Autodesk Inventor part; units mm, degrees
ref_plane "YZ Plane" through (0, 0, 0) normal (1, 0, 0) x (0, 1, 0)
ref_plane "XZ Plane" through (0, 0, 0) normal (0, 1, 0) x (-1, 0, 0)
ref_plane "XY Plane" through (0, 0, 0) normal (0, 0, 1) x (1, 0, 0)
sketch "Sketch1" plane through (0, 0, 0) normal (1, 0, 0) x (0, 1, 0)
  line L0 (0, 0) -> (50.8, 0)
  line L1 (50.8, 0) -> (50.8, -25.4)
  line L2 (50.8, -25.4) -> (0, -25.4)
  line L3 (0, -25.4) -> (0, 0)
  line L4 (47.625, -22.225) -> (47.625, -3.175)
  line L5 (47.625, -3.175) -> (3.175, -3.175)
  line L6 (3.175, -3.175) -> (3.175, -22.225)
  line L7 (3.175, -22.225) -> (47.625, -22.225)
  dimension "d0" = 50.8
  dimension "d1" = 25.4
  dimension "d2" = 3.175
extrude "Extrusion1" add sketch "Sketch1" along normal blind 177.8
sketch "Sketch2" plane through (0, 0, 0) normal (0, 0, 1) x (1, 0, 0)
  line L0 (0, 0) -> (0, 50.8)
  circle A0 centre (81.28, 25.4) radius 14.2875
  line L1 (151.13, 25.4) -> (175.8823, 25.4) construction
  line L2 (81.28, 25.4) -> (106.68, 25.4) construction
  circle A1 centre (99.2405, 43.3605) radius 2.0193
  circle A2 centre (63.3195, 7.4395) radius 2.0193
  circle A3 centre (63.3195, 7.4395) radius 2.0193
  circle A4 centre (99.2405, 43.3605) radius 2.0193
  dimension "d5" = 81.28
  dimension "d6" = 28.575
  dimension "d19" = 4.0386
  dimension "d20" = 4.0386
extrude "Extrusion2" cut sketch "Sketch2" against normal blind 25.4 contours A0
sketch "Sketch3" plane through (177.8, 0, 0) normal (1, 0, 0) x (0, 0, -1)
  line L0 (0, 50.8) -> (0, 0)
  line L1 (25.4, 0) -> (25.4, 50.8)
  line L2 (0, 0) -> (25.4, 0)
  line L3 (25.4, 0) -> (25.4, 50.8)
  line L4 (25.4, 50.8) -> (0, 50.8)
  line L5 (0, 50.8) -> (0, 0)
  line L6 (3.175, 3.175) -> (3.175, 47.625)
  line L7 (3.175, 47.625) -> (22.225, 47.625)
  line L8 (3.175, 3.175) -> (22.225, 3.175)
  line L9 (22.225, 3.175) -> (22.225, 47.625)
  line L10 (22.225, 47.625) -> (3.175, 47.625)
  line L11 (3.175, 47.625) -> (3.175, 3.175)
extrude "Extrusion3" add sketch "Sketch3" along normal blind 228.6
sketch "Sketch4" plane through (0, 0, 0) normal (0, 0, 1) x (1, 0, 0)
  circle A0 centre (81.28, 25.4) radius 14.2875
  line L0 (0, 50.8) -> (406.4, 50.8)
  line L1 (81.28, 25.4) -> (106.68, 25.4) construction
  circle A1 centre (99.2405, 43.3605) radius 2.0193
  circle A2 centre (63.3195, 7.4395) radius 2.0193
  point P0 (0, 0)
  dimension "d22" = 4.0386
  dimension "d23" = 4.0386
extrude "Extrusion4" cut sketch "Sketch4" against normal blind 228.6 contours A1 | A2
properties part number "liftCimBar" material "Aluminum 6061"
Can you work these out from the model? Positions are in its coordinate system, mm. A direction names the side the tool comes from. Coordinates: 2 decimals unless noted, no trailing zeros. Order: outer loops, then holes, each group sorted by start corner. A loop starts at its lowest first (then second) coordinate and runs counter-clockwise, first axis right, second up.
1. If we section it at A-A (y = 25.4): Please give me the cut outline in (x, z) (1 decimal), then the cut area to 3 significant figures.
2. If we section it at C-C (z = -10): Please give me the cut outline in (x, y) (3 decimals).
3. I'm going to push a flat-ended pin straight in: pin 1 (2.5 mm diameter, centred on x = 63.32, y = 7.44, fed in from -Z). Where does the tip first touch, or does it pass through?
4. Thinking about a two-plate mould opening in Z: for faces 3 (the face through (406.4, 24, -2)), 4 (the face through (200, 25, -25.4)), 5 (the face through (200, 26, 0)), 6 (the face through (200, 47.625, -13)), which applies, +Z half, -Z half, draft (parallel to the pull), parting line (faces both ways), or undercut?
5. I need wall thicknesses on line 1 (Y direction, x = 162.5, z = -18.75) (3 decimals); line 2 (Z direction, x = 247, y = 20) (3 decimals); line 3 (Y direction, x = 81.28, z = -0.9). Which ranges of each line are inside material? Lowest first, please.
6. If we section it at B-B (x = 81.28): Please give me the cut outline in (y, z) (1 decimal), then the cut area to 3 significant figures.
7. For faces 1 (the face through (67.006, 26.028, -23.79)), 2 (the face through (200, 25, -3.175)), which set-ups out of +Z, -Z, +X, -X, +Y, -Y let a thin tool reach every point of the face, with its end or its side?
Entries:
1. outline: (0, -25.4) - (67, -25.4) - (67, -22.2) - (0, -22.2) - close; (0, -3.2) - (67, -3.2) - (67, 0) - (0, 0) - close; (95.6, -25.4) - (406.4, -25.4) - (406.4, -22.2) - (95.6, -22.2) - close; (95.6, -3.2) - (406.4, -3.2) - (406.4, 0) - (95.6, 0) - close
1. area: 2,400 mm2
2. outline: (0, 0) - (406.4, 0) - (406.4, 3.175) - (0, 3.175) - close; (0, 47.625) - (406.4, 47.625) - (406.4, 50.8) - (0, 50.8) - close
3. pin 1: passes through
4. face 3: draft
4. face 4: -Z half
4. face 5: +Z half
4. face 6: undercut
5. line 1: y = 0 to 3.175, 47.625 to 50.8
5. line 2: z = -25.4 to -22.225, -3.175 to 0
5. line 3: y = 0 to 11.11, 39.69 to 50.8
6. outline: (0, -25.4) - (11.1, -25.4) - (11.1, -22.2) - (3.2, -22.2) - (3.2, -3.2) - (11.1, -3.2) - (11.1, 0) - (0, 0) - close; (39.7, -25.4) - (50.8, -25.4) - (50.8, 0) - (39.7, 0) - (39.7, -3.2) - (47.6, -3.2) - (47.6, -22.2) - (39.7, -22.2) - close
6. area: 262 mm2
7. face 1: +Z, -Z
7. face 2: +X, -X
